from build123d import *

# Parameters (mm, degrees)
BOSS_EXTRUDE1_DEPTH = 2
BOSS_EXTRUDE2_DEPTH = 55
BOSS_EXTRUDE3_DEPTH = 2
SKETCH4_R           = 4
CUT_EXTRUDE1_DEPTH  = 60


with BuildPart() as part:
    # Sketch1 → Boss-Extrude1 (new body)
    with BuildSketch(Plane.XY):
        with BuildLine():
            Line((-17, 0), (0, 0))
            Line((0, 0), (0, 17))
            Line((0, 17), (0, 34))
            Line((0, 34), (-17, 34))
            Line((-17, 34), (-34, 34))
            Line((-34, 34), (-34, 17))
            ThreePointArc((-34, 17), (-29.02081528, 4.97918472), (-17, 0))
        make_face()
    extrude(amount=BOSS_EXTRUDE1_DEPTH)

    # Sketch2 → Boss-Extrude2 (add)
    with BuildSketch(Plane.XY.offset(2)):
        with BuildLine():
            Line((-17, 0), (0, 0))
            Line((0, 0), (0, 1.5))
            Line((0, 1.5), (-17, 1.5))
            ThreePointArc((-17, 1.5), (-27.960155108, 6.039844892), (-32.5, 17))
            Line((-32.5, 17), (-32.5, 34))
            Line((-32.5, 34), (-34, 34))
            Line((-34, 34), (-34, 17))
            ThreePointArc((-34, 17), (-29.02081528, 4.97918472), (-17, 0))
        make_face()
    extrude(amount=BOSS_EXTRUDE2_DEPTH)

    # Sketch3 → Boss-Extrude3 (add)
    with BuildSketch(Plane.XY.offset(57)):
        with BuildLine():
            Line((0, 0), (0, 1.5))
            Line((0, 1.5), (0, 34))
            Line((0, 34), (-32.5, 34))
            Line((-32.5, 34), (-34, 34))
            Line((-34, 34), (-34, 17))
            ThreePointArc((-34, 17), (-29.02081528, 4.97918472), (-17, 0))
            Line((-17, 0), (0, 0))
        make_face()
    extrude(amount=BOSS_EXTRUDE3_DEPTH)

    # Sketch4 → Cut-Extrude1 (cut, through all)
    with BuildSketch(Plane.XY.offset(59)):
        with Locations((-17, 17)):
            Circle(SKETCH4_R)
    extrude(amount=-CUT_EXTRUDE1_DEPTH, mode=Mode.SUBTRACT)


solid = part.part
Source: CAD feature listing. Evaluate the final solid. Frame: model axes, mm. A direction names the side the tool comes from. Give positions to 0.01 mm unless a question says otherwise; leave off trailing zeros. Write each loop counter-clockwise with the first axis right and the second up, starting at its lowest first coordinate (ties: lowest second). Pieces come first, ordered by that corner, then holes. Notation, with made-up numbers: M 2,-21.5 L 14,-21.5 A29 cw 14,7.5 Z; hole C 27,49.25 d6. An arc over 180 degrees is marked long. Return JSON: item names as keys, results as strings. Group by question number.
1) First-contact query: pin 1 Ø1 at (y, z) = (26, 52) entering from +X; pin 2 Ø1 at (x, z) = (-4.5, 49.5) entering from -Y; pin 3 Ø6 at (y, z) = (14.5, 23.5) entering from +X; pin 4 Ø10 at (y, z) = (3.5, 43) entering from -X. Flat tips, straight axial feed; report the tip coordinate or a pass-through.
2) Draft query along Z for faces 1 (the face through (-29.15, 5.11, 29.09)), 2 (the face through (-32.5, 25, 29)), 3 (the face through (-13, 21, 0)). Return one class per face: released by +Z, released by -Z, zero draft, split by the parting line, or undercut.
3) Cut plane A-A, the plane z = 52. Output: boundary loops of the cut face in (x, y), then the cut area to 3 significant figures.
4) Set-up query: faces 4 (the face through (-8, 1.5, 29)), 5 (the face through (-19.95, 19.7, 58.01)). Return all of +Z, -Z, +X, -X, +Y, -Y with unobstructed straight access to the full face (end or side cutting, diameter ignored); none if empty.
5) Cut plane C-C, the plane y = 15. Output: boundary loops of the cut face in (x, z), then the cut area to 3 significant figures.
6) Ray query, L1, parallel to Z at x = -8, y = 3; L2, parallel to Y at x = -17, z = 1; L3, parallel to X at y = 30.5, z = 33.5. Return the intervals inside material, ascending.
7) Cut plane B-B, the plane x = -3. Output: boundary loops of the cut face in (y, z), then the cut area to 4 significant figures.
Data:
{
 "1": {"pin 1": "stops at x = -32.5", "pin 2": "stops at y = 0", "pin 3": "stops at x = -31.49", "pin 4": "stops at x = -31.72"},
 "2": {"face 1": "zero draft", "face 2": "undercut", "face 3": "released by -Z"},
 "3": {"outline": "M -34,17 A17 ccw -17,0 L 0,0 L 0,1.5 L -17,1.5 A15.5 cw -32.5,17 L -32.5,34 L -34,34 Z", "area": "89.3 mm²"},
 "4": {"face 4": "+X, +Y", "face 5": "+Z, -Z"},
 "5": {"outline": "M -33.88,0 L -20.46,0 L -20.46,2 L -32.37,2 L -32.37,57 L -20.46,57 L -20.46,59 L -33.88,59 Z; M -13.54,0 L 0,0 L 0,2 L -13.54,2 Z; M -13.54,57 L 0,57 L 0,59 L -13.54,59 Z", "area": "191 mm²"},
 "6": {"L1": "z = 0 to 2, 57 to 59", "L2": "y = 0 to 13, 21 to 34", "L3": "x = -34 to -32.5"},
 "7": {"outline": "M 0,0 L 34,0 L 34,2 L 1.5,2 L 1.5,57 L 34,57 L 34,59 L 0,59 Z", "area": "218.5 mm²"}
}
